Autodesk Inventor part; units mm, degrees
ref_plane "YZ Plane" through (0, 0, 0) normal (1, 0, 0) x (0, 1, 0)
ref_plane "XZ Plane" through (0, 0, 0) normal (0, 1, 0) x (-1, 0, 0)
ref_plane "XY Plane" through (0, 0, 0) normal (0, 0, 1) x (1, 0, 0)
sketch "Sketch1" plane through (0, 0, 0) normal (0, 1, 0) x (-1, 0, 0)
  point P0 (0, 0)
sketch "Sketch2" plane through (0, 0, 0) normal (0, 1, 0) x (-1, 0, 0)
  line L0 (0, 0) -> (-16.129, 0)
  line L1 (-16.129, 0) -> (-16.129, 28.194)
  line L2 (-16.129, 28.194) -> (0, 28.194)
  line L3 (0, 28.194) -> (0, 0)
  circle A0 centre (-8.0645, 20.9296) radius 2.9464
  point P0 (-8.0645, 28.194)
  dimension "d0" = 16.129
  dimension "d1" = 28.194
  dimension "d3" = 5.8928
  dimension "d4" = 7.2644
extrude "Extrusion1" add sketch "Sketch2" along normal blind 2.0066
sketch "Sketch3" plane through (0, 0, 0) normal (0, -1, 0) x (1, 0, 0)
  line L0 (16.129, 0) -> (0, 0)
  line L1 (0, 0) -> (16.129, 0)
  line L2 (16.129, 0) -> (16.129, 2.0066)
  line L3 (16.129, 2.0066) -> (0, 2.0066)
  line L4 (0, 2.0066) -> (0, 0)
  point P0 (8.0645, 2.0066)
  dimension "d7" = 2.0066
extrude "Extrusion2" add sketch "Sketch3" against normal blind 27.94
fillet "Fillet1" radius 6.35 2 edges at (16.129, 1.0033, 28.194) (0, 1.0033, 28.194)
sketch "Sketch4" plane through (0, 2.0066, 2.0066) normal (0, 0, 1) x (1, 0, 0)
  circle A0 centre (8.0645, 18.669) radius 2.9464
  line L0 (0, 25.9334) -> (16.129, 25.9334)
  point P0 (0, -2.0066)
  point P1 (8.0645, 25.9334)
  dimension "d11" = 5.8928
  dimension "d12" = 7.2644
fillet "Fillet2" radius 6.35 2 edges at (0, 27.94, 1.0033) (16.129, 27.94, 1.0033)
extrude "Extrusion3" cut sketch "Sketch4" against normal blind 2.0066
fillet "Fillet3" radius 0.254 20 edges at (14.2691, 2.0066, 26.3341) (8.0645, 2.0066, 28.194) (1.8599, 2.0066, 26.3341) (0, 2.0066, 11.9253) (16.129, 2.0066, 11.9253) (14.2691, 0, 26.3341) (8.0645, 0, 28.194) (1.8599, 0, 26.3341) (0, 0, 10.922) (16.129, 0, 10.922) (14.2691, 26.0801, 2.0066) (8.0645, 27.94, 2.0066) (1.8599, 26.0801, 2.0066) (0, 11.7983, 2.0066) (16.129, 11.7983, 2.0066) (14.2691, 26.0801, 0) (8.0645, 27.94, 0) (1.8599, 26.0801, 0) (0, 10.795, 0) (16.129, 10.795, 0)
properties part number "Right Angle"
Read the model definition and answer for the solid it produces. Units are mm, in the model's axes. A direction names the side the tool comes from. Give positions to 0.01 mm unless a question says otherwise; leave off trailing zeros. Write each loop counter-clockwise with the first axis right and the second up, starting at its lowest first coordinate (ties: lowest second). Pieces come first, ordered by that corner, then holes. Notation, with made-up numbers: (16.5, -23) - (23.5, -23) arc R17 cw to (23.5, -17) - close; hole circle Ø1 at (49.25, 76). An arc over 180 degrees is marked (long way). Write item = value, one per line. Start each with the question number.
Item 1: Find section A-A (y = 11.25). Give the vertices of the cut face in (x, z) (3 decimals), then the cut area to 3 significant figures.
Item 2: Find section B-B (x = 7.5). Give the vertices of the cut face in (y, z), then the cut area to 3 significant figures.
Item 3: Find section C-C (z = 20.25). Give the vertices of the cut face in (x, y) (3 decimals).
Item 4: The mould has two halves that part along X. Classify faces 1 (the cylindrical face through (9.65, 23.16, 1.02)), 2 (the flat face through (8, 15, 2.007)), 3 (the flat face through (16.129, 6, 1)), 4 (the cylindrical face through (1.811, 1.014, 26.284)): +X half, -X half, draft (parallel to the pull), parting line (faces both ways), or undercut.
Item 5: Each of these flat-tipped pins is pushed along its axis until it touches: P1, Ø8, axis at x = 10.5, y = 12.5, coming from the +Z side; P2, Ø3, axis at x = 12, z = 5, coming from the +Y side. Where does it stop, or does it pass through?
Item 6: Find the intervals of material crossed by probe 1 along Z at (x, y) = (15, 16.5), in increasing order. Write a range as [from, to].
Item 7: A tool of negligible diameter and unlimited length cuts with its end or side. For faces 5 (the flat face through (8, 2.007, 15)), 6 (the flat face through (8, 1, 28.194)), from which of +Z, -Z, +X, -X, +Y, -Y can it reach the whole face along a straight path? Write none if from no direction.
Response:
q1.outline = (0, 0.254) arc R0.254 ccw to (0.254, 0) - (15.875, 0) arc R0.254 ccw to (16.129, 0.254) - (16.129, 1.753) arc R0.254 ccw to (15.875, 2.007) - (0.254, 2.007) arc R0.254 ccw to (0, 1.753) - close
q1.area = 32.3 mm²
q2.outline = (0, 0) - (17.78, 0) - (17.78, 2.01) - (2.01, 2.01) - (2.01, 18.04) - (0, 18.04) - close; (0, 23.82) - (2.01, 23.82) - (2.01, 27.94) arc R0.25 ccw to (1.75, 28.19) - (0.25, 28.19) arc R0.25 ccw to (0, 27.94) - close; (23.57, 0) - (27.69, 0) arc R0.25 ccw to (27.94, 0.25) - (27.94, 1.75) arc R0.25 ccw to (27.69, 2.01) - (23.57, 2.01) - close
q2.area = 85.3 mm²
q3.outline = (0, 0.254) arc R0.254 ccw to (0.254, 0) - (5.198, 0) - (5.198, 2.007) - (0.254, 2.007) arc R0.254 ccw to (0, 1.753) - close; (10.931, 0) - (15.875, 0) arc R0.254 ccw to (16.129, 0.254) - (16.129, 1.753) arc R0.254 ccw to (15.875, 2.007) - (10.931, 2.007) - close
q4.face_1 = undercut
q4.face_2 = draft
q4.face_3 = +X half
q4.face_4 = -X half
q5.P1 = 2.01
q5.P2 = 2.01
q6.probe_1 = [0, 2.01]
q7.face_5 = +Z, +X, -X, +Y
q7.face_6 = +Z, +X, -X, +Y, -Y
